from build123d import *

# Parameters (mm, degrees)
BOSS_EXTRUDE3_DEPTH = 3
SKETCH3_W           = 5
SKETCH3_H           = 2.5
CUT_EXTRUDE1_DEPTH  = 3


with BuildPart() as part:
    # Sketch2 → Boss-Extrude3 (new body)
    with BuildSketch(Plane.XY):
        with BuildLine():
            Line((0.1, 0), (1, 0))
            Line((1, 0), (7.900193166, -0.429508089))
            ThreePointArc((7.900193166, -0.429508089), (7.968947639, -0.463133775), (7.993787443, -0.53552748))
            Line((7.993787443, -0.53552748), (7.968937216, -0.934754817))
            Line((7.968937216, -0.934754817), (0.984453593, -0.5))
            Line((0.984453593, -0.5), (0, -0.5))
            Line((0, -0.5), (0, -0.1))
            ThreePointArc((0, -0.1), (0.029289322, -0.029289322), (0.1, 0))
        make_face()
    extrude(amount=BOSS_EXTRUDE3_DEPTH)

    # Sketch3 → Cut-Extrude1 (cut)
    with BuildSketch(Plane(origin=(0.003859586, 0.062005564, 0), x_dir=(0.998068341, -0.062125569, 0), z_dir=(0.062125569, 0.998068341, 0))):
        with Locations((4.317122221, -1.500788282)):
            Rectangle(SKETCH3_W, SKETCH3_H)
    extrude(amount=-CUT_EXTRUDE1_DEPTH, mode=Mode.SUBTRACT)


solid = part.part
Can you work these out from the model? Positions are in its coordinate system, mm. A direction names the side the tool comes from. Coordinates: 2 decimals unless noted, no trailing zeros. Loops run counter-clockwise (first coordinate to the right, second up) from the corner with the lowest first, then second, coordinate; pieces in that order, holes last. Notation, with made-up numbers: M -38,10.5 L -29,10.5 A20 ccw -29,29.5 Z; hole C -31.5,-25.75 d4. An arc over 180 degrees is marked long. Return JSON: item names as keys, results as strings. Group by question number.
Item 1: Imagine slicing it at B-B (x = 4.25). Please give me the cut outline in (y, z), and give its area (3 significant figures).
Item 2: If I drill on L1, parallel to Z at x = 3.25, y = -0.55; L2, parallel to Y at x = 0.5, z = 1.75; L3, parallel to Y at x = 7.25, z = 1.55, over which ranges is the centre line in solid material (lowest first)? Write a range as from..to.
Item 3: I'm going to push a flat-ended pin straight in: pin 1 Ø0.8 at (x, z) = (0.5, 2) entering from -Y. Where does the tip first touch, or does it pass through?
Item 4: Thinking about a two-plate mould opening in Z: for faces 1 (the flat face through (0.5, -0.5, 1.5)), 2 (the flat face through (4.1, -0.5, 0)), 3 (the flat face through (4.3, -0.5, 2.751)), which applies, released by +Z, released by -Z, zero draft, split by the parting line, or undercut?
Item 5: On a 3-axis mill with a long thin cutter (end or side, diameter ignored), from which of +Z, -Z, +X, -X, +Y, -Y can I reach the whole of each face in a straight line? I mean faces 4 (the flat face through (0.5, 0, 1.5)), 5 (the flat face through (4.3, -0.5, 0.251)). Say none if no direction works.
Item 6: Imagine slicing it at D-D (x = 0.75). Please give me the cut outline in (y, z), and give its area (3 significant figures).
Item 7: Imagine slicing it at A-A (z = 2.05). Please give me the cut outline in (x, y), and give its area (3 significant figures).
Item 8: Imagine slicing it at C-C (y = -0.7). Please give me the cut outline in (x, z), and give its area (3 significant figures).
Verdict:
{
 "1": {"outline": "M -0.7,0 L -0.2,0 L -0.2,0.25 L -0.7,0.25 Z; M -0.7,2.75 L -0.2,2.75 L -0.2,3 L -0.7,3 Z", "area": "0.250 mm^2"},
 "2": {"L1": "z = 0..0.25, 2.75..3", "L2": "y = -0.5..0", "L3": "y = -0.89..-0.39"},
 "3": {"pin 1": "stops at y = -0.5"},
 "4": {"face 1": "zero draft", "face 2": "released by -Z", "face 3": "undercut"},
 "5": {"face 4": "+Z, -Z, +X, -X, +Y", "face 5": "+Y, -Y"},
 "6": {"outline": "M -0.5,0 L 0,0 L 0,3 L -0.5,3 Z", "area": "1.50 mm^2"},
 "7": {"outline": "M 0,-0.5 L 0.98,-0.5 L 1.79,-0.55 L 1.82,-0.05 L 1,0 L 0.1,0 A0.1 ccw 0,-0.1 Z; M 6.78,-0.86 L 7.97,-0.93 L 7.99,-0.54 A0.1 ccw 7.9,-0.43 L 6.81,-0.36 Z", "area": "1.49 mm^2"},
 "8": {"outline": "M 4.2,0 L 7.98,0 L 7.98,3 L 4.2,3 L 4.2,2.75 L 6.79,2.75 L 6.79,0.25 L 4.2,0.25 Z", "area": "4.89 mm^2"}
}
